```python
from build123d import *

# Parameters (mm, degrees)
PAD006_DEPTH = 13
PAD007_DEPTH = 6.5
SKETCH005_R  = 1.05
PAD005_DEPTH = 1.65


with BuildPart() as connectorbody:
    # Sketch006 → Pad006 (new body)
    with BuildSketch(Plane.XZ):
        with BuildLine():
            Line((-14, 6), (14, 6))
            ThreePointArc((16, 4), (15.414214, 5.414214), (14, 6))
            Line((16, 4), (16, -4))
            ThreePointArc((14, -6), (15.414214, -5.414214), (16, -4))
            Line((14, -6), (-14, -6))
            ThreePointArc((-16, -4), (-15.414214, -5.414214), (-14, -6))
            Line((-16, -4), (-16, 4))
            ThreePointArc((-14, 6), (-15.414214, 5.414214), (-16, 4))
        make_face()
    extrude(amount=PAD006_DEPTH)


with BuildPart() as connectorbody_1:
    # Body005 placement: moved
    add(connectorbody.part.moved(Location((0, 45, 7.65))))


with BuildPart() as usbbody:
    # Sketch007 → Pad007 (new body)
    with BuildSketch(Plane.XZ):
        with BuildLine():
            ThreePointArc((-3, 1.5), (-4.5, 0), (-3, -1.5))
            Line((-3, -1.5), (3, -1.5))
            ThreePointArc((3, -1.5), (4.5, 0), (3, 1.5))
            Line((-3, 1.5), (3, 1.5))
        make_face()
    extrude(amount=PAD007_DEPTH)


with BuildPart() as usbbody_1:
    # Body006 placement: moved
    add(usbbody.part.moved(Location((-20, -38.7, 3.15))))


with BuildPart() as boardpart:
    # Sketch005 → Pad005 (new body)
    with BuildSketch(Plane.XY):
        with BuildLine():
            Line((-32, 45), (32, 45))
            ThreePointArc((35, 42), (34.12132, 44.12132), (32, 45))
            Line((35, 42), (35, -42))
            ThreePointArc((32, -45), (34.12132, -44.12132), (35, -42))
            Line((32, -45), (-32, -45))
            ThreePointArc((-35, -42), (-34.12132, -44.12132), (-32, -45))
            Line((-35, -42), (-35, 42))
            ThreePointArc((-32, 45), (-34.12132, 44.12132), (-35, 42))
        make_face()
        with Locations((-32, -42)):
            Circle(SKETCH005_R, mode=Mode.SUBTRACT)
        with Locations((32, -42)):
            Circle(SKETCH005_R, mode=Mode.SUBTRACT)
        with Locations((32, 42)):
            Circle(SKETCH005_R, mode=Mode.SUBTRACT)
        with Locations((-32, 42)):
            Circle(SKETCH005_R, mode=Mode.SUBTRACT)
    extrude(amount=PAD005_DEPTH)

    # Fusion: union ConnectorBody, UsbBody
    add(connectorbody_1.part)
    add(usbbody_1.part)


with BuildPart() as boardpart_1:
    # Fusion placement: moved
    add(boardpart.part.moved(Location((0, 0, 4.05))))


solid = boardpart_1.part
```
For this review, take the finished solid that the model builds, in its own axes (mm). A direction names the side the tool comes from. Coordinates: 2 decimals unless noted, no trailing zeros. Write each loop counter-clockwise with the first axis right and the second up, starting at its lowest first coordinate (ties: lowest second). Pieces come first, ordered by that corner, then holes.
(1) Tool access review of faces 4 (the face through (32.97, 41.6, 4.86)), 5 (the face through (16, 39, 12)): name each direction out of +Z, -Z, +X, -X, +Y, -Y from which nothing blocks a thin tool from reaching the whole face with its end or side.
(2) For pin 1 Ø1.7 at (x, y) = (-32, -42) entering from +Z; pin 2 Ø3.5 at (x, z) = (2, 10) entering from -Y; pin 3 Ø2.5 at (y, z) = (40.5, 12) entering from +X; pin 4 Ø0.8 at (x, z) = (-12.5, 4.5) entering from -Y, all flat-tipped, find the tip position at first contact; note any pin that passes through.
(3) Add section C-C on z = 12. Give the boundary of the cut face in (x, y), then the cut area to 3 significant figures.
(4) The part is to be moulded in two halves that separate along Z. For faces 1 (the face through (0, 1, 4.05)), 2 (the face through (15.4, 38.59, 6.27)), 3 (the face through (-20, -38.7, 7)), say which applies: +Z half, -Z half, draft (parallel to the pull), parting line (faces both ways), or undercut.
(5) Wall thickness on probe 1 along Y at (x, z) = (-32, 5.25); probe 2 along Y at (x, z) = (-10.5, 6.75); probe 3 along Z at (x, y) = (1, -10): over which ranges is each line inside the solid? List them lowest first.
(6) Add section A-A on y = 38. Give the boundary of the cut face in (x, z), then the cut area to 3 significant figures.
(7) Add section B-B on x = -29. Give the boundary of the cut face in (y, z), then the cut area to 4 significant figures.
Answer sheet:
1. face 4: +Z, -Z
1. face 5: +Z, +X, +Y, -Y
2. pin 1: passes through
2. pin 2: stops at y = 32
2. pin 3: stops at x = 16
2. pin 4: stops at y = -45
3. outline: (-16, 32) - (16, 32) - (16, 45) - (-16, 45) - close
3. area: 416 mm2
4. face 1: -Z half
4. face 2: undercut
4. face 3: draft
5. probe 1: y = -45 to -43.05, -40.95 to 40.95, 43.05 to 45
5. probe 2: y = 32 to 45
5. probe 3: z = 4.05 to 5.7
6. outline: (-35, 4.05) - (35, 4.05) - (35, 5.7) - (14, 5.7) arc R2 ccw to (16, 7.7) - (16, 15.7) arc R2 ccw to (14, 17.7) - (-14, 17.7) arc R2 ccw to (-16, 15.7) - (-16, 7.7) arc R2 ccw to (-14, 5.7) - (-35, 5.7) - close
6. area: 496 mm2
7. outline: (-45, 4.05) - (45, 4.05) - (45, 5.7) - (-45, 5.7) - close
7. area: 148.5 mm2
